```python
from build123d import *

# Parameters (mm, degrees)
EXTRUDE_1_DEPTH     = 85
CUT_EXTRUDE_1_DEPTH = 26
SKETCH_3_W          = 32
SKETCH_3_H          = 21
CUT_EXTRUDE_2_DEPTH = 10


with BuildPart() as part:
    # Эскиз1 → Вытянуть-Тонкостенный1 (new body)
    with BuildSketch(Plane(origin=(0, 0, 0), x_dir=(0, 0, -1), z_dir=(1, 0, 0))):
        Polygon((0, 25), (0, 0), (25, 0), (25, 4), (4, 4), (4, 25), align=None)
    extrude(amount=EXTRUDE_1_DEPTH)

    # Эскиз2 → Вырез-Вытянуть1 (cut, through all)
    with BuildSketch(Plane.XY):
        Polygon((0, 0), (0, 25), (25, 25), align=None)
        Polygon((60, 25), (85, 25), (85, 0), align=None)
    extrude(amount=-CUT_EXTRUDE_1_DEPTH, mode=Mode.SUBTRACT)

    # Эскиз3 → Вырез-Вытянуть2 (cut)
    with BuildSketch(Plane.XZ):
        with Locations((16, -14.5)):
            Rectangle(SKETCH_3_W, SKETCH_3_H)
    extrude(amount=-CUT_EXTRUDE_2_DEPTH, mode=Mode.SUBTRACT)


solid = part.part
```
Input: part model. Units: mm. Frame: model coordinates. A direction names the side the tool comes from. Round coordinates to 2 decimals unless told otherwise and drop trailing zeros. Loops run counter-clockwise (first coordinate to the right, second up) from the corner with the lowest first, then second, coordinate; pieces in that order, holes last.
1) Pin query (flat end, axial travel): pin 1 (4 mm diameter, centred on x = 38.5, y = 11, fed in from -Z); pin 2 (1.2 mm diameter, centred on y = 1.5, z = -12, fed in from -X); pin 3 (2 mm diameter, centred on y = 6.5, z = -22.5, fed in from -X). Return the tip coordinate at first contact, or that it passes through.
Ans:
pin 1: stops at z = -4
pin 2: stops at x = 32
pin 3: passes through
2) Set-up query: faces 1 (the flat face through (56, 4, -15)), 2 (the flat face through (32, 2, -15)), 3 (the flat face through (51, 0, -12)). Return all of +Z, -Z, +X, -X, +Y, -Y with unobstructed straight access to the full face (end or side cutting, diameter ignored); none if empty.
Ans:
face 1: -Z, +X, -X, +Y
face 2: -Z, -X, +Y, -Y
face 3: +Z, -Z, +X, -X, -Y
3) Section query C-C on y = 13. Return the cut outline in (x, z), plus the area to 3 significant figures.
Ans:
outline: (13, -4) - (72, -4) - (72, 0) - (13, 0) - close
area: 236 mm2
4) Section query A-A on x = 73. Return the cut outline in (y, z), plus the area to 3 significant figures.
Ans:
outline: (0, -25) - (4, -25) - (4, -4) - (12, -4) - (12, 0) - (0, 0) - close
area: 132 mm2
5) Section query D-D on x = 54. Return the cut outline in (y, z), plus the area to 3 significant figures.
Ans:
outline: (0, -25) - (4, -25) - (4, -4) - (25, -4) - (25, 0) - (0, 0) - close
area: 184 mm2
6) Section query B-B on z = -21. Return the cut outline in (x, y), plus the area to 3 significant figures.
Ans:
outline: (32, 0) - (85, 0) - (81, 4) - (32, 4) - close
area: 204 mm2
7) Material intervals for line 1 (Z direction, x = 23.5, y = 12); line 2 (Y direction, x = 46, z = -12.5); line 3 (X direction, y = 2, z = -15.25), sorted ascending.
Ans:
line 1: z = -4 to 0
line 2: y = 0 to 4
line 3: x = 32 to 83
